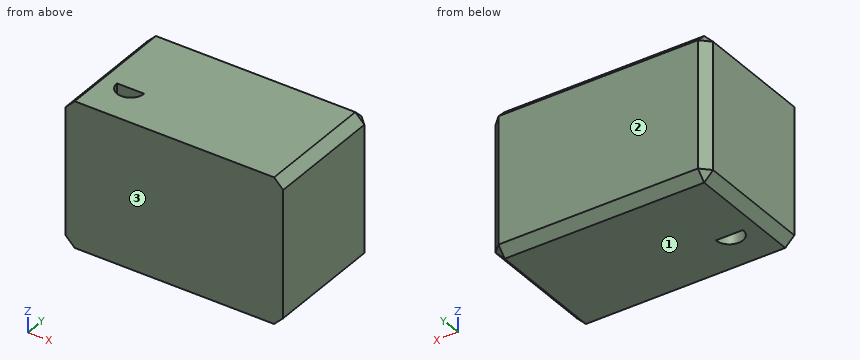
from build123d import *

# Parameters (mm, degrees)
SKETCH1_W           = 120
SKETCH1_H           = 70
BOSS_EXTRUDE3_DEPTH = 80
CHAMFER2_SIZE       = 5
CUT_EXTRUDE1_DEPTH  = 161.312195419


with BuildPart() as part:
    # Sketch1 → Boss-Extrude3 (new body)
    with BuildSketch(Plane.XY):
        with Locations((60, 35)):
            Rectangle(SKETCH1_W, SKETCH1_H)
    extrude(amount=-BOSS_EXTRUDE3_DEPTH)

    # Chamfer2
    chamfer2_edges = [part.edges().sort_by_distance(p)[0] for p in [
        (60, 70, -80),
        (0, 35, -80),
        (0, 35, 0),
        (60, 70, 0),
        (120, 35, 0),
        (0, 70, -40),
        (120, 70, -40),
        (120, 35, -80),
    ]]
    chamfer(chamfer2_edges, length=CHAMFER2_SIZE)

    # Sketch5 → Cut-Extrude1 (cut, through all)
    with BuildSketch(Plane.XY):
        with BuildLine():
            Line((12.5, 23), (27.5, 23))
            ThreePointArc((27.5, 23), (20, 15.5), (12.5, 23))
        make_face()
    extrude(amount=-CUT_EXTRUDE1_DEPTH, mode=Mode.SUBTRACT)


solid = part.part
Read the model definition and answer for the solid it produces. Units are mm, in the model's axes. Face numbers are marked on the shaded views. Round coordinates to 2 decimals unless told otherwise and drop trailing zeros. Loops run counter-clockwise (first coordinate to the right, second up) from the corner with the lowest first, then second, coordinate; pieces in that order, holes last.
Q1. Consider probe 1 along Y at (x, z) = (24.5, -20); probe 2 along X at (y, z) = (21.5, -45.5); probe 3 along Y at (x, z) = (24, -39.5). Determine where each line is inside the solid, lowest interval first.
Q2. Determine the mould class of the marked faces 1, 2 and 3 for opening direction Y: released by +Y, released by -Y, zero draft, split by the parting line, or undercut.
Q3. Section A-A on x = 20 is taken. Write down the section's boundary in (y, z).
Output:
1. probe 1: y = 0 to 17, 23 to 70
1. probe 2: x = 0 to 12.65, 27.35 to 120
1. probe 3: y = 0 to 16.66, 23 to 70
2. face 1: zero draft
2. face 2: released by +Y
2. face 3: released by -Y
3. outline: (0, -80) - (15.5, -80) - (15.5, 0) - (0, 0) - close; (23, -80) - (65, -80) - (70, -75) - (70, -5) - (65, 0) - (23, 0) - close
